```python
from build123d import *

# Parameters (mm, degrees)
SKETCH3_W               = 40
SKETCH3_H               = 43
BOSS_EXTRUDE1_DEPTH     = 3
SKETCH4_W               = 40
SKETCH4_H               = 3
BOSS_EXTRUDE2_DEPTH     = 24
SKETCH6_R               = 20
BOSS_EXTRUDE3_DEPTH     = 3
SKETCH7_R               = 1.5
CUT_EXTRUDE1_DEPTH      = 8
FILLET1_R               = 3
SKETCH8_R               = 2
CUT_EXTRUDE2_DEPTH      = 8
MIRROR3_COPY_1_SKETCH_R = 2
MIRROR3_COPY_1_DEPTH    = 8
FILLET2_R               = 3
CUT_EXTRUDE3_DEPTH      = 8


with BuildPart() as part:
    # Sketch3 → Boss-Extrude1 (new body)
    with BuildSketch(Plane(origin=(0, 0, 0), x_dir=(1, 0, 0), z_dir=(0, 1, 0))):
        Rectangle(SKETCH3_W, SKETCH3_H)
    extrude(amount=BOSS_EXTRUDE1_DEPTH)

    # Sketch4 → Boss-Extrude2 (add)
    with BuildSketch(Plane(origin=(0, 3, 0), x_dir=(1, 0, 0), z_dir=(0, 1, 0))):
        with Locations((0, 20)):
            Rectangle(SKETCH4_W, SKETCH4_H)
    extrude(amount=BOSS_EXTRUDE2_DEPTH)

    # Sketch6 → Boss-Extrude3 (add)
    with BuildSketch(Plane.XY.offset(-18.5)):
        with Locations((0, 27)):
            Circle(SKETCH6_R)
    extrude(amount=-BOSS_EXTRUDE3_DEPTH)

    # Sketch7 → Cut-Extrude1 (cut)
    with BuildSketch(Plane.XY.offset(-18.5)):
        with Locations((7.65, 40.296356644)):
            Circle(SKETCH7_R)
        with Locations((15.34, 27)):
            Circle(SKETCH7_R)
        with Locations((6.432903226, 13.074004305)):
            Circle(SKETCH7_R)
    cut_extrude1 = extrude(amount=-CUT_EXTRUDE1_DEPTH, mode=Mode.SUBTRACT)

    # Mirror1: Cut-Extrude1 across plane
    add(cut_extrude1.mirror(Plane(origin=(0, 0, 0), x_dir=(0, 0, 1), z_dir=(1, 0, 0))), mode=Mode.SUBTRACT)

    # Fillet1
    fillet1_edges = [part.edges().sort_by_distance(p)[0] for p in [
        (0, 0, -21.5),
    ]]
    fillet(fillet1_edges, radius=FILLET1_R)

    # Sketch8 → Cut-Extrude2 (cut)
    with BuildSketch(Plane(origin=(0, 3, 0), x_dir=(1, 0, 0), z_dir=(0, 1, 0))):
        with Locations((-15, 12)):
            Circle(SKETCH8_R)
    cut_extrude2 = extrude(amount=-CUT_EXTRUDE2_DEPTH, mode=Mode.SUBTRACT)

    # Mirror2: Cut-Extrude2 across plane
    add(cut_extrude2.mirror(Plane(origin=(0, 0, 0), x_dir=(0, 0, 1), z_dir=(1, 0, 0))), mode=Mode.SUBTRACT)

    # Mirror3: Cut-Extrude2 across plane
    add(cut_extrude2.mirror(Plane.XY), mode=Mode.SUBTRACT)

    # Mirror3 copy 1 sketch → Mirror3 copy 1 (cut)
    with BuildSketch(Plane(origin=(0, 3, 0), x_dir=(-1, 0, 0), z_dir=(0, 1, 0))):
        with Locations((-15, 12)):
            Circle(MIRROR3_COPY_1_SKETCH_R)
    extrude(amount=-MIRROR3_COPY_1_DEPTH, mode=Mode.SUBTRACT)

    # Fillet2
    fillet2_edges = [part.edges().sort_by_distance(p)[0] for p in [
        (20, 1.5, 21.5),
        (-20, 1.5, 21.5),
    ]]
    fillet(fillet2_edges, radius=FILLET2_R)

    # Sketch9 → Cut-Extrude3 (cut)
    with BuildSketch(Plane.XY.offset(-18.5)):
        with BuildLine():
            Line((6, 34.5), (6, 19.5))
            ThreePointArc((6, 19.5), (0, 13.5), (-6, 19.5))
            Line((-6, 19.5), (-6, 34.5))
            ThreePointArc((-6, 34.5), (0, 40.5), (6, 34.5))
        make_face()
    extrude(amount=-CUT_EXTRUDE3_DEPTH, mode=Mode.SUBTRACT)


solid = part.part
```
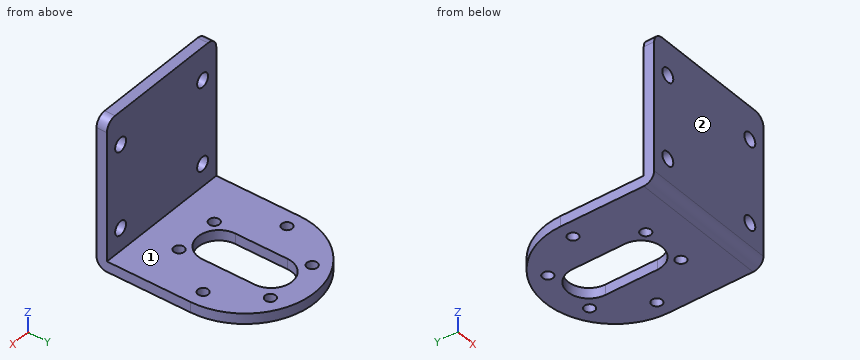
Verification items for the finished model (mm, model axes). Face numbers are marked on the shaded views. A direction names the side the tool comes from. Round coordinates to 2 decimals unless told otherwise and drop trailing zeros. Write each loop counter-clockwise with the first axis right and the second up, starting at its lowest first coordinate (ties: lowest second). Pieces come first, ordered by that corner, then holes.
1. Gauge pin test, flat ends, axial feed: P1, Ø4, axis at x = 7.65, y = 40.3, coming from the -Z side; P2, Ø4.5, axis at x = -15, z = 12, coming from the +Y side; P3, Ø20, axis at x = -10, y = 27, coming from the +Z side. Record the tip position at first contact, or that the pin passes through.
2. Section check A-A on z = 12. Enter the section's corners in (x, y).
3. Section check C-C on y = 21. Enter the section's corners in (x, z).
4. Section check D-D on x = -15. Enter the section's corners in (y, z).
5. Section check B-B on x = 0. Enter the section's corners in (y, z), plus the area to 3 significant figures.
6. Scan lines: L1, parallel to X at y = 0.95, z = -12; L2, parallel to Z at x = -15, y = 1.05; L3, parallel to Y at x = -7, z = -19 (1 decimal). Record each from-to range of solid material in increasing order.
7. Access from +Z, -Z, +X, -X, +Y, -Y to the whole of each face (thin tool, end or side, straight path). Record for the marked faces 1 and 2.
Answer:
1. P1: stops at z = -21.5
1. P2: stops at y = 3
1. P3: stops at z = -18.5
2. outline: (-20, 0) - (-17, 0) - (-17, 3) - (-20, 3) - close; (-13, 0) - (13, 0) - (13, 3) - (-13, 3) - close; (17, 0) - (20, 0) - (20, 3) - (17, 3) - close
3. outline: (-20, -21.5) - (-6, -21.5) - (-6, -18.5) - (-20, -18.5) - close; (6, -21.5) - (20, -21.5) - (20, -18.5) - (6, -18.5) - close
4. outline: (0, -18.5) arc R3 ccw to (3, -21.5) - (25.54, -21.5) - (25.54, -18.5) - (3, -18.5) - (3, -14) - (0, -14) - close; (0, -10) - (3, -10) - (3, 10) - (0, 10) - close; (0, 14) - (3, 14) - (3, 21.5) - (0, 21.5) - close; (28.46, -21.5) - (40.23, -21.5) - (40.23, -18.5) - (28.46, -18.5) - close
5. outline: (0, -18.5) arc R3 ccw to (3, -21.5) - (13.5, -21.5) - (13.5, -18.5) - (3, -18.5) - (3, 21.5) - (0, 21.5) - close; (40.5, -21.5) - (47, -21.5) - (47, -18.5) - (40.5, -18.5) - close
5. area: 178 mm2
6. L1: x = -20 to -17, -13 to 13, 17 to 20
6. L2: z = -20.78 to -14, -10 to 10, 14 to 21.5
6. L3: y = 0 to 11.7, 14.5 to 38.9, 41.6 to 45.7
7. face 1: +Z, +X, -X, +Y
7. face 2: +Z, -Z, +X, -X, -Y
